The model under review builds one solid part; all positions refer to its coordinate system, in mm. Give positions to 0.01 mm unless a question says otherwise; leave off trailing zeros. Order: outer loops, then holes, each group sorted by start corner. A loop starts at its lowest first (then second) coordinate and runs counter-clockwise, first axis right, second up. Notation, with made-up numbers: (-3.5, 75.5) - (36.5, 75.5) arc R15 ccw to (36.5, 80.5) - close; hole circle Ø4 at (59.25, 2.5). An arc over 180 degrees is marked (long way). Use CSV: the item, a comma, the result in double quotes. Start each with the question number.
1. Draft analysis for pull direction Y (two halves, no side actions). For faces 1 (the cylindrical face through (-0.111, 13.524, 8.801)), 2 (the cylindrical face through (-1.72, -7.75, 3.54)), 3 (the flat face through (-14.288, 0, 3)), state which applies: released by +Y, released by -Y, zero draft, split by the parting line, or undercut.
2. To check wall thickness, follow line 1 (X direction, y = -8.25, z = 0.5); line 2 (Y direction, x = -1.5, z = 6.5); line 3 (X direction, y = 5, z = 8.75). State the ranges of each line that lie inside material, in increasing order. Write a range as [from, to].
3. Take a section at D-D, the plane z = 8. State the section outline as (x, y) points, then the cut area to 3 significant figures.
4. For pin 1 (2 mm diameter, centred on x = 10.5, z = 4, fed in from +Y), flat-tipped, find the tip position at first contact; note if it passes through.
5. Take a section at A-A, the plane x = 0. State the section outline as (y, z) points (1 decimal), then the cut area to 3 significant figures.
```python
from build123d import *

# Parameters (mm, degrees)
F0_W     = 28.575
F0_H     = 28.575
F1_DEPTH = 9.525
F2_R     = 7.9375
F3_DEPTH = 9.526
F4_R     = 6.35
F5_R     = 2.54


with BuildPart() as f1:
    # F0 (on Top) → F1 (new body)
    with BuildSketch(Plane.XY):
        Rectangle(F0_W, F0_H)
    extrude(amount=F1_DEPTH)

    # F2 (on face) → F3 (cut, through all)
    with BuildSketch(Plane.XY.offset(9.525)):
        Circle(F2_R)
    extrude(amount=-F3_DEPTH, mode=Mode.SUBTRACT)

    # F4
    f4_edges = [f1.edges().sort_by_distance(p)[0] for p in [
        (-14.2875, -14.2875, 4.7625),
        (-14.2875, 14.2875, 4.7625),
        (14.2875, -14.2875, 4.7625),
        (14.2875, 14.2875, 4.7625),
    ]]
    fillet(f4_edges, radius=F4_R)

    # F5
    f5_edges = [f1.edges().sort_by_distance(p)[0] for p in [
        (-7.9375, 0, 9.525),
        (0, -14.2875, 9.525),
    ]]
    fillet(f5_edges, radius=F5_R)


solid = f1.part
```
Determined:
1,face 1,"released by +Y"
1,face 2,"undercut"
1,face 3,"zero draft"
2,line 1,"x = [-14.28, 14.28]"
2,line 2,"y = [-14.29, -7.79], [7.79, 14.29]"
2,line 3,"x = [-13.57, -7.06], [7.06, 13.57]"
3,outline,"(-14.08, -7.94) arc R6.14 ccw to (-7.94, -14.08) - (7.94, -14.08) arc R6.14 ccw to (14.08, -7.94) - (14.08, 7.94) arc R6.14 ccw to (7.94, 14.08) - (-7.94, 14.08) arc R6.14 ccw to (-14.08, 7.94) - close; hole circle Ø16.3 at (0, 0)"
3,area,"552 mm²"
4,pin 1,"stops at y = 14.09"
5,outline,"(-14.3, 0) - (-7.9, 0) - (-7.9, 7) arc R2.5 ccw to (-10.5, 9.5) - (-11.7, 9.5) arc R2.5 ccw to (-14.3, 7) - close; (7.9, 0) - (14.3, 0) - (14.3, 7) arc R2.5 ccw to (11.7, 9.5) - (10.5, 9.5) arc R2.5 ccw to (7.9, 7) - close"
5,area,"115 mm²"
